Input: part model. Units: mm. Frame: model coordinates. Face numbers are marked on the shaded views. A direction names the side the tool comes from. Coordinates: 2 decimals unless noted, no trailing zeros. Order: outer loops, then holes, each group sorted by start corner. A loop starts at its lowest first (then second) coordinate and runs counter-clockwise, first axis right, second up. Notation, with made-up numbers: (38, 72) - (89, 72) arc R11 ccw to (89, 92) - close; hole circle Ø6 at (19, 25). An arc over 180 degrees is marked (long way). Answer as CSV lines item,"result". Start each with the question number.
Item 1: Draft query along Z for the marked faces 1, 2 and 3. Return one class per face: +Z half, -Z half, draft (parallel to the pull), parting line (faces both ways), or undercut.
Item 2: Material intervals for line 1 along Z through (x, y) = (33.9, 7.75); line 2 along Y through (x, z) = (31, -2.75); line 3 along X through (y, z) = (-12.4, -8), sorted ascending.
Item 3: Section D-D (z = -7.25). State how many separate pieces and enclosed holes the cut face has, and give its area (3 significant figures).
Item 4: Access query for the marked faces 4 and 5. Directions: +Z, -Z, +X, -X, +Y, -Y. A direction counts if a zero-diameter tool reaches every point of the face in a straight line with its end or side. Return the directions, or none.
Item 5: Section C-C (y = 7.75). Output: boundary loops of the cut face in (x, z).
Item 6: Section B-B (x = 34.5). Output: boundary loops of the cut face in (y, z).
Item 7: Section A-A (y = -2.25). Output: boundary loops of the cut face in (x, z), and give its area (3 significant figures).
Item 8: First-contact query: pin 1 (1.2 mm diameter, centred on x = 24.5, z = -8.5, fed in from -Y); pin 2 (4 mm diameter, centred on y = -1, z = 6, fed in from -X); pin 3 (1.2 mm diameter, centred on x = 23.5, z = -7, fed in from +Y). Flat tips, straight axial feed; report the tip coordinate or a pass-through.
from build123d import *

# Parameters (mm, degrees)
SKETCH_1_R          = 1.25
EXTRUDE_1_DEPTH     = 14.5
SKETCH_2_R          = 33
CUT_EXTRUDE_1_DEPTH = 11.75
SKETCH_3_R          = 0.75
SKETCH_3_W          = 9
SKETCH_3_H          = 21
CUT_EXTRUDE_2_DEPTH = 25.169333236
EXTRUDE_START       = 2
SKETCH_4_R          = 1.5
SKETCH_4_R_2        = 0.75
EXTRUDE_2_DEPTH     = 2
FILLET_1_R          = 2
FILLET_2_R          = 3
CHAMFER_1_SIZE      = 1
SKETCH_5_R          = 1.95
CUT_EXTRUDE_3_DEPTH = 1


with BuildPart() as part:
    # Эскиз1 → Бобышка-Вытянуть1 (new, symmetric)
    with BuildSketch(Plane(origin=(0, 0, 0), x_dir=(1, 0, 0), z_dir=(0, 1, 0))):
        with BuildLine():
            Line((34, 13), (19.685438565, 13))
            Line((19.685438565, 13), (19.685438565, 3.5))
            Line((19.685438565, 3.5), (25, 3.5))
            ThreePointArc((25, 3.5), (27.474873734, 2.474873734), (28.5, 0))
            ThreePointArc((28.5, 0), (27.474873734, -2.474873734), (25, -3.5))
            Line((25, -3.5), (19.685438565, -3.5))
            Line((19.685438565, -3.5), (19.685438565, -13))
            Line((19.685438565, -13), (34, -13))
            Line((34, -13), (34, 13))
        make_face()
        with Locations(Location((23.685438565, -8, 0), (0, 0, 90))):
            Circle(SKETCH_1_R, mode=Mode.SUBTRACT)
        with Locations(Location((23.685438565, 8, 0), (0, 0, 90))):
            Circle(SKETCH_1_R, mode=Mode.SUBTRACT)
    extrude(amount=EXTRUDE_1_DEPTH, both=True)

    # Эскиз2 → Вырез-Вытянуть1 (cut, symmetric)
    with BuildSketch(Plane(origin=(0, 0, 0), x_dir=(1, 0, 0), z_dir=(0, 1, 0))):
        Circle(SKETCH_2_R)
    extrude(amount=CUT_EXTRUDE_1_DEPTH, both=True, mode=Mode.SUBTRACT)

    # Эскиз3 → Вырез-Вытянуть2 (cut, through all)
    with BuildSketch(Plane(origin=(34, 0, 0), x_dir=(0, 0, -1), z_dir=(1, 0, 0))):
        with Locations((7, 7.75)):
            Circle(SKETCH_3_R)
        with Locations((7, -7.75)):
            Circle(SKETCH_3_R)
        with Locations((-2.5, 0)):
            Rectangle(SKETCH_3_W, SKETCH_3_H)
    extrude(amount=-CUT_EXTRUDE_2_DEPTH, mode=Mode.SUBTRACT)

    # Эскиз4 → Бобышка-Вытянуть2 (add)
    # profile 1 of 2: a face of its own
    with BuildSketch(Plane(origin=(34, 0, 0), x_dir=(0, 0, -1), z_dir=(1, 0, 0)).offset(EXTRUDE_START)):
        with Locations((7, 7.75)):
            Circle(SKETCH_4_R)
        with Locations((7, 7.75)):
            Circle(SKETCH_4_R_2, mode=Mode.SUBTRACT)
    # profile 2 of 2: a face of its own
    with BuildSketch(Plane(origin=(34, 0, 0), x_dir=(0, 0, -1), z_dir=(1, 0, 0)).offset(EXTRUDE_START)):
        with Locations((7, -7.75)):
            Circle(SKETCH_4_R)
        with Locations((7, -7.75)):
            Circle(SKETCH_4_R_2, mode=Mode.SUBTRACT)
    extrude(amount=-EXTRUDE_2_DEPTH)

    # Скругление1
    fillet_1_edges = [part.edges().sort_by_distance(p)[0] for p in [
        (33.469669092, 10.5, -2),
        (33.469669092, -10.5, -2),
        (33.124515497, -10.5, 7),
        (33.124515497, 10.5, 7),
    ]]
    fillet(fillet_1_edges, radius=FILLET_1_R)

    # Скругление2
    fillet_2_edges = [part.edges().sort_by_distance(p)[0] for p in [
        (19.685438565, 13.125, -3.5),
        (19.685438565, 13.125, -13),
        (19.685438565, 13.125, 13),
        (19.685438565, 13.125, 3.5),
        (19.685438565, -13.125, -3.5),
        (19.685438565, -13.125, -13),
        (19.685438565, -13.125, 13),
        (19.685438565, -13.125, 3.5),
    ]]
    fillet(fillet_2_edges, radius=FILLET_2_R)

    # Фаска1
    chamfer_1_edges = [part.edges().sort_by_distance(p)[0] for p in [
        (19.685438565, -14.5, -8.25),
        (23.842719282, 14.5, 3.5),
        (23.842719282, -14.5, -3.5),
        (28.342719282, -14.5, -13),
        (28.342719282, -14.5, 13),
        (19.685438565, -14.5, 8.25),
        (20.564118221, -14.5, 12.121320344),
        (20.564118221, -14.5, 4.378679656),
        (20.564118221, -14.5, -4.378679656),
        (20.564118221, -14.5, -12.121320344),
        (28.342719282, 14.5, -13),
        (28.342719282, 14.5, 13),
        (19.685438565, 14.5, -8.25),
        (19.685438565, 14.5, 8.25),
        (20.564118221, 14.5, 12.121320344),
        (20.564118221, 14.5, 4.378679656),
        (20.564118221, 14.5, -4.378679656),
        (20.564118221, 14.5, -12.121320344),
        (23.842719282, -14.5, 3.5),
        (28.5, -14.5, 0),
        (23.842719282, 14.5, -3.5),
        (28.5, 14.5, 0),
    ]]
    chamfer(chamfer_1_edges, length=CHAMFER_1_SIZE)

    # Эскиз5 → Вырез-Вытянуть3 (cut)
    with BuildSketch(Plane(origin=(0, 14.5, 0), x_dir=(1, 0, 0), z_dir=(0, 1, 0))):
        with Locations(Location((23.685438565, -8, 0), (0, 0, 270))):
            Circle(SKETCH_5_R)
        with Locations(Location((23.685438565, 8, 0), (0, 0, 270))):
            Circle(SKETCH_5_R)
    cut_extrude_3 = extrude(amount=-CUT_EXTRUDE_3_DEPTH, mode=Mode.SUBTRACT)

    # Зеркальное отражение1: Вырез-Вытянуть3 across plane
    add(cut_extrude_3.mirror(Plane.ZX), mode=Mode.SUBTRACT)


solid = part.part
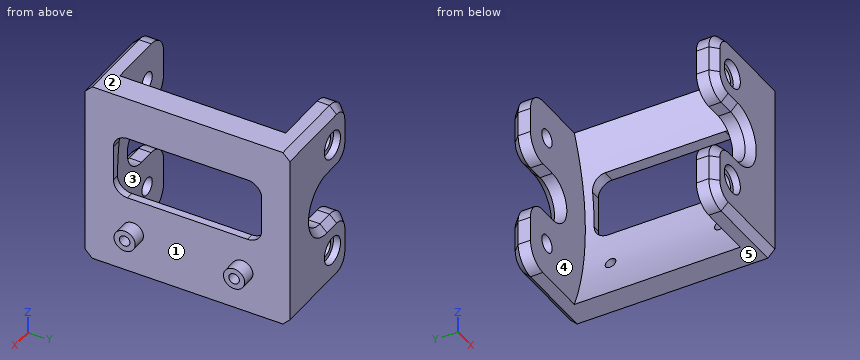
Determined:
1,face 1,"draft"
1,face 2,"+Z half"
1,face 3,"undercut"
2,line 1,"z = -13 to -7.75, -6.25 to -2, 7 to 13"
2,line 2,"y = -14.5 to -11.75, 11.75 to 14.5"
2,line 3,"x = 19.69 to 22.44, 24.94 to 34"
3,separate pieces,"5"
3,enclosed holes,"0"
3,area,"107 mm^2"
4,face 4,"-X"
4,face 5,"-Z, +X, -X, +Y, -Y"
5,outline,"(30.33, -13) - (34, -13) - (34, -8.5) - (36, -8.5) - (36, -7.75) - (32.08, -7.75) arc R33 cw to start; (30.33, 13) arc R33 cw to (32.25, 7) - (34, 7) - (34, 13) - close; (32.4, -6.25) - (36, -6.25) - (36, -5.5) - (34, -5.5) - (34, -2) - (32.94, -2) arc R33 cw to start"
6,outline,"circle Ø3 at (-7.75, -7); circle Ø3 at (7.75, -7); hole circle Ø1.5 at (-7.75, -7); hole circle Ø1.5 at (7.75, -7)"
7,outline,"(30.33, -13) - (34, -13) - (34, -2) - (32.94, -2) arc R33 cw to start; (30.33, 13) arc R33 cw to (32.25, 7) - (34, 7) - (34, 13) - close"
7,area,"38.0 mm^2"
8,pin 1,"stops at y = -13.5"
8,pin 2,"stops at x = 32.02"
8,pin 3,"stops at y = 13.5"
